from build123d import *

# Parameters (mm, degrees)
F0_R     = 19.05
F1_DEPTH = 3.5
F3_DEPTH = 5.334
F5_DEPTH = 25.4


# Not quite as in the source:
# - a feature names something its author has since deleted; it is built from what else it names


with BuildPart() as f1:
    # F0 (on Top) → F1 (new body)
    with BuildSketch(Plane.XY):
        Circle(F0_R)
    extrude(amount=F1_DEPTH)

    # F2 (on face) → F3 (cut)
    with BuildSketch(Plane.XY.offset(3.5)):
        with BuildLine():
            Line((0, -3.175), (0.5430206191, -3.175))
            ThreePointArc((0.5430206191, -3.175), (2.1121063082, -2.6323908231), (3.0107980648, -1.2363937796))
            add(Edge.make_bspline(
                [(6.35, 3.175), (6.1354222845, 2.6541048515), (5.9660194487, 1.4359488031), (3.5744657813, 0.5479613391), (3.1233221277, -0.7746591325), (3.0107980648, -1.2363937796)],
                knots=[0, 0, 0, 0, 0.2694475223, 0.6162953248, 0.7809262502, 0.7809262502, 0.7809262502, 0.7809262502], degree=3))
            Line((6.35, 3.175), (6.35, 9.525))
            ThreePointArc((6.35, 9.525), (4.4901280605, 14.0151280605), (0, 15.875))
            Line((0, 15.875), (0, -3.175))
        make_face()
        with BuildLine():
            Line((-0.5430206191, -3.175), (0, -3.175))
            Line((0, -3.175), (0, 15.875))
            ThreePointArc((0, 15.875), (-4.4901280605, 14.0151280605), (-6.35, 9.525))
            Line((-6.35, 9.525), (-6.35, 3.175))
            add(Edge.make_bspline(
                [(-6.35, 3.175), (-6.1354222845, 2.6541048515), (-5.9660194487, 1.4359488031), (-3.5744657813, 0.5479613391), (-3.1233221277, -0.7746591325), (-3.0107980648, -1.2363937796)],
                knots=[0, 0, 0, 0, 0.2694475223, 0.6162953248, 0.7809262502, 0.7809262502, 0.7809262502, 0.7809262502], degree=3))
            ThreePointArc((-3.0107980648, -1.2363937796), (-2.1121063082, -2.6323908231), (-0.5430206191, -3.175))
        make_face()
    extrude(amount=-F3_DEPTH, mode=Mode.SUBTRACT)

    # F4 (on face) → F5 (cut)
    with BuildSketch(Plane.XY.offset(3.5)):
        with BuildLine():
            Line((-12.2672579939, -3.0629981272), (-11.9385578066, -1.8362723278))
            Line((-11.9385578066, -1.8362723278), (-9.8138063951, -2.4055977526))
            ThreePointArc((-9.8138063951, -2.4055977526), (-10.3831318199, -2.0768975654), (-10.7118320072, -1.5075721405))
            ThreePointArc((-10.7118320072, -1.5075721405), (-12.1993062273, -0.5933281371), (-13.1939593601, -2.0282799825))
            ThreePointArc((-13.1939593601, -2.0282799825), (-13.1812823619, -2.2901216321), (-13.2226351142, -2.5489878245))
            Line((-13.2226351142, -2.5489878245), (-13.3516440016, -3.030455547))
            ThreePointArc((-13.3516440016, -3.030455547), (-13.4452645639, -3.2753166219), (-13.5871639911, -3.4957396431))
            ThreePointArc((-13.5871639911, -3.4957396431), (-13.4432450328, -5.2357709608), (-11.697932569, -5.1877495387))
            ThreePointArc((-11.697932569, -5.1877495387), (-11.1286071442, -4.8590493514), (-10.4712067697, -4.8590493514))
            Line((-10.4712067697, -4.8590493514), (-12.5959581812, -4.2897239266))
            Line((-12.5959581812, -4.2897239266), (-12.2672579939, -3.0629981272))
        make_face()
        Polygon((-9.8138063951, -2.4055977526), (-11.9385578066, -1.8362723278), (-12.2672579939, -3.0629981272), (-2.4534515988, -5.6925996254), (0, -5.0351992509), align=None)
        Polygon((-2.4534515988, -5.6925996254), (-12.2672579939, -3.0629981272), (-12.5959581812, -4.2897239266), (-10.4712067697, -4.8590493514), (-4.9069031975, -6.35), align=None)
        with BuildLine():
            Line((9.8138063951, -2.4055977526), (0, -5.0351992509))
            Line((0, -5.0351992509), (2.4534515988, -5.6925996254))
            Line((2.4534515988, -5.6925996254), (4.9069031975, -6.35))
            Line((4.9069031975, -6.35), (10.4712067697, -4.8590493514))
            ThreePointArc((10.4712067697, -4.8590493514), (11.1286071442, -4.8590493514), (11.697932569, -5.1877495387))
            ThreePointArc((11.697932569, -5.1877495387), (13.4432450328, -5.2357709608), (13.5871639911, -3.4957396431))
            ThreePointArc((13.5871639911, -3.4957396431), (13.4452645639, -3.2753166219), (13.3516440016, -3.030455547))
            Line((13.3516440016, -3.030455547), (13.2226351142, -2.5489878245))
            ThreePointArc((13.2226351142, -2.5489878245), (13.1812823619, -2.2901216321), (13.1939593601, -2.0282799825))
            ThreePointArc((13.1939593601, -2.0282799825), (12.1993062273, -0.5933281371), (10.7118320072, -1.5075721405))
            ThreePointArc((10.7118320072, -1.5075721405), (10.3831318199, -2.0768975654), (9.8138063951, -2.4055977526))
        make_face()
        Polygon((0, -6.35), (0, -5.0351992509), (-2.4534515988, -5.6925996254), align=None)
        Polygon((2.4534515988, -5.6925996254), (0, -5.0351992509), (0, -6.35), align=None)
        Polygon((0, -6.35), (-2.4534515988, -5.6925996254), (-4.9069031975, -6.35), (-2.4534515988, -7.0074003746), align=None)
        Polygon((4.9069031975, -6.35), (2.4534515988, -5.6925996254), (0, -6.35), align=None)
        Polygon((4.9069031975, -6.35), (0, -6.35), (2.4534515988, -7.0074003746), align=None)
        Polygon((2.4534515988, -7.0074003746), (0, -6.35), (-2.4534515988, -7.0074003746), (0, -7.6648007491), align=None)
        Polygon((-2.4534515988, -7.0074003746), (-4.9069031975, -6.35), (-10.4712067697, -7.8409506486), (-12.5959581812, -8.4102760734), (-12.2672579939, -9.6370018728), align=None)
        Polygon((10.4712067697, -7.8409506486), (4.9069031975, -6.35), (2.4534515988, -7.0074003746), (12.2672579939, -9.6370018728), (12.5959581812, -8.4102760734), align=None)
        Polygon((12.2672579939, -9.6370018728), (2.4534515988, -7.0074003746), (0, -7.6648007491), (9.8138063951, -10.2944022474), (11.9385578066, -10.8637276722), align=None)
        Polygon((0, -7.6648007491), (-2.4534515988, -7.0074003746), (-12.2672579939, -9.6370018728), (-11.9385578066, -10.8637276722), (-9.8138063951, -10.2944022474), align=None)
        with BuildLine():
            Line((-12.5959581812, -8.4102760734), (-10.4712067697, -7.8409506486))
            ThreePointArc((-10.4712067697, -7.8409506486), (-11.1286071442, -7.8409506486), (-11.697932569, -7.5122504613))
            ThreePointArc((-11.697932569, -7.5122504613), (-13.4432450328, -7.4642290392), (-13.5871639911, -9.2042603569))
            ThreePointArc((-13.5871639911, -9.2042603569), (-13.4452645639, -9.4246833781), (-13.3516440016, -9.669544453))
            Line((-13.3516440016, -9.669544453), (-13.2226351142, -10.1510121755))
            ThreePointArc((-13.2226351142, -10.1510121755), (-13.1812823619, -10.4098783679), (-13.1939593601, -10.6717200175))
            ThreePointArc((-13.1939593601, -10.6717200175), (-12.1993062273, -12.1066718629), (-10.7118320072, -11.1924278595))
            ThreePointArc((-10.7118320072, -11.1924278595), (-10.3831318199, -10.6231024346), (-9.8138063951, -10.2944022474))
            Line((-9.8138063951, -10.2944022474), (-11.9385578066, -10.8637276722))
            Line((-11.9385578066, -10.8637276722), (-12.2672579939, -9.6370018728))
            Line((-12.2672579939, -9.6370018728), (-12.5959581812, -8.4102760734))
        make_face()
        with BuildLine():
            ThreePointArc((11.697932569, -7.5122504613), (11.1286071442, -7.8409506486), (10.4712067697, -7.8409506486))
            Line((10.4712067697, -7.8409506486), (12.5959581812, -8.4102760734))
            Line((12.5959581812, -8.4102760734), (12.2672579939, -9.6370018728))
            Line((12.2672579939, -9.6370018728), (11.9385578066, -10.8637276722))
            Line((11.9385578066, -10.8637276722), (9.8138063951, -10.2944022474))
            ThreePointArc((9.8138063951, -10.2944022474), (10.3831318199, -10.6231024346), (10.7118320072, -11.1924278595))
            ThreePointArc((10.7118320072, -11.1924278595), (12.1993062273, -12.1066718629), (13.1939593601, -10.6717200175))
            ThreePointArc((13.1939593601, -10.6717200175), (13.1812823619, -10.4098783679), (13.2226351142, -10.1510121755))
            Line((13.2226351142, -10.1510121755), (13.3516440016, -9.669544453))
            ThreePointArc((13.3516440016, -9.669544453), (13.4452645639, -9.4246833781), (13.5871639911, -9.2042603569))
            ThreePointArc((13.5871639911, -9.2042603569), (13.4432450328, -7.4642290392), (11.697932569, -7.5122504613))
        make_face()
    extrude(amount=-F5_DEPTH, mode=Mode.SUBTRACT)


solid = f1.part
Part model, mm, in its own coordinate system. A direction names the side the tool comes from. Coordinates: 2 decimals unless noted, no trailing zeros. Write each loop counter-clockwise with the first axis right and the second up, starting at its lowest first coordinate (ties: lowest second). Pieces come first, ordered by that corner, then holes. Notation, with made-up numbers: (29.25, 60) - (33.25, 60) arc R22 cw to (33.25, 73) - close; hole circle Ø3 at (18.5, 29). An arc over 180 degrees is marked (long way). Put each result on its own line as item: value.
1. Probe line 1 along Y through (x, z) = (6.5, 3); line 2 along Y through (x, z) = (0.5, 1.4) (3 decimals); line 3 along X through (y, z) = (-1.5, 2.4). List the from-to ranges inside material, lowest first. Write a range as [from, to].
Final values:
line 1: y = [-17.91, -9.41], [-6.78, -5.92], [-3.29, 17.91]
line 2: y = [-19.043, -7.799], [-4.901, -3.175], [15.855, 19.043]
line 3: x = [-18.99, -13.16], [-10.71, -2.93], [2.93, 10.71], [13.16, 18.99]
2. Band-saw the part on B-B (y = 7.5). Write the cut outline in (x, z).
Final values:
outline: (-17.51, 0) - (-6.35, 0) - (-6.35, 3.5) - (-17.51, 3.5) - close; (6.35, 0) - (17.51, 0) - (17.51, 3.5) - (6.35, 3.5) - close
3. Band-saw the part on D-D (y = -14). Write the cut outline in (x, z).
Final values:
outline: (-12.92, 0) - (12.92, 0) - (12.92, 3.5) - (-12.92, 3.5) - close
4. 3-axis set-ups, long thin cutter, end or side, ignore diameter. For faces 4 (the flat face through (-7.7, -7.1, 1.8)), 5 (the flat face through (4, 0, 3.5)): which of +Z, -Z, +X, -X, +Y, -Y reach the whole face in a straight line?
Final values:
face 4: +Z, -Z
face 5: +Z, +X, -X, +Y, -Y
5. Two-plate mould, pull along Y, no slides. Class faces 1 (the flat face through (4, 0, 0)), 2 (the cylindrical face through (-15.12, -11.59, 1.73)), 3 (the cylindrical face through (2.09, -2.65, 1.77)): +Y half, -Y half, draft (parallel to the pull), parting line (faces both ways), or undercut.
Final values:
face 1: draft
face 2: parting line
face 3: undercut
6. Band-saw the part on C-C (z = 1.3). Give the number of separate pieces and of enclosed holes in the cut face, then the cut area to 3 significant figures.
Final values:
separate pieces: 1
enclosed holes: 2
area: 797 mm²
7. Flat gauge pins, fed straight in: pin 1 Ø1 at (y, z) = (-5.5, 2) entering from +X; pin 2 Ø1 at (y, z) = (-4, 0.5) entering from +X; pin 3 Ø0.5 at (x, z) = (0, 1.5) entering from +Y; pin 4 Ø2 at (x, y) = (-1, -10.5) entering from -Z. Where does each tip first touch, or does it go through?
Final values:
pin 1: stops at x = 18.38
pin 2: stops at x = 18.73
pin 3: stops at y = 19.05
pin 4: stops at z = 0
8. Band-saw the part on A-A (y = -4). Write the cut outline in (x, z), then the cut area to 3 significant figures.
Final values:
outline: (-18.63, 0) - (-13.83, 0) - (-13.83, 3.5) - (-18.63, 3.5) - close; (-3.86, 0) - (3.86, 0) - (3.86, 3.5) - (-3.86, 3.5) - close; (13.83, 0) - (18.63, 0) - (18.63, 3.5) - (13.83, 3.5) - close
area: 60.6 mm²
